```python
from build123d import *

# Parameters (mm, degrees)
CROQUIS1_W                 = 73.8
CROQUIS1_H                 = 70
SALIENTE_EXTRUIR1_DEPTH    = 1.9
CROQUIS2_R                 = 6.35
CORTAR_EXTRUIR1_DEPTH      = 1
CORTAR_EXTRUIR1_DEPTH_BACK = 2.9


with BuildPart() as part:
    # Croquis1 → Saliente-Extruir1 (new body)
    with BuildSketch(Plane(origin=(0, 0, 0), x_dir=(1, 0, 0), z_dir=(0, 1, 0))):
        Rectangle(CROQUIS1_W, CROQUIS1_H)
    extrude(amount=SALIENTE_EXTRUIR1_DEPTH)

    # Croquis2 → Cortar-Extruir1 (cut, two sides)
    with BuildSketch(Plane(origin=(0, 1.9, 0), x_dir=(1, 0, 0), z_dir=(0, 1, 0))) as cortar_extruir1_sk:
        with Locations((0, -20)):
            Circle(CROQUIS2_R)
    extrude(amount=CORTAR_EXTRUIR1_DEPTH, mode=Mode.SUBTRACT)
    extrude(cortar_extruir1_sk.sketch, amount=-CORTAR_EXTRUIR1_DEPTH_BACK, mode=Mode.SUBTRACT)


solid = part.part
```
Work out the finished part from the listing and answer in its coordinate system (mm). Coordinates: 2 decimals unless noted, no trailing zeros. Loops run counter-clockwise (first coordinate to the right, second up) from the corner with the lowest first, then second, coordinate; pieces in that order, holes last.
1) Section C-C (y = 1.5) is taken. Give the vertices of the cut face in (x, z).
Results:
outline: (-36.9, -35) - (36.9, -35) - (36.9, 35) - (-36.9, 35) - close; hole circle Ø12.7 at (0, 20)
2) For a pull along X with two mould halves and no side action, classify faces 1 (the flat face through (-1, 1.9, 0)), 2 (the cylindrical face through (-1.38, 0.96, 26.2)), 3 (the flat face through (-36.9, 1, 0)) as +X half, -X half, draft (parallel to the pull), parting line (faces both ways), or undercut.
Results:
face 1: draft
face 2: undercut
face 3: -X half
3) Section B-B (x = 0) is taken. Give the vertices of the cut face in (y, z).
Results:
outline: (0, -35) - (1.9, -35) - (1.9, 13.65) - (0, 13.65) - close; (0, 26.35) - (1.9, 26.35) - (1.9, 35) - (0, 35) - close
4) Section A-A (z = 20) is taken. Give the vertices of the cut face in (x, y).
Results:
outline: (-36.9, 0) - (-6.35, 0) - (-6.35, 1.9) - (-36.9, 1.9) - close; (6.35, 0) - (36.9, 0) - (36.9, 1.9) - (6.35, 1.9) - close
5) Consider probe 1 along X at (y, z) = (1.45, 20); probe 2 along Z at (x, y) = (0, 0.9). Determine where each line is inside the solid, lowest interval first.
Results:
probe 1: x = -36.9 to -6.35, 6.35 to 36.9
probe 2: z = -35 to 13.65, 26.35 to 35
